Check sheet for the modelled part. Datum: model origin and axes. Units: mm. Face numbers are marked on the shaded views. Round coordinates to 2 decimals unless told otherwise and drop trailing zeros. Loops run counter-clockwise (first coordinate to the right, second up) from the corner with the lowest first, then second, coordinate; pieces in that order, holes last. Notation, with made-up numbers: M 76.5,11.25 L 122.5,11.25 A16 cw 122.5,36.25 Z; hole C -28.75,-26 d2. An arc over 180 degrees is marked long. One line per question, with ' | ' between items. Start each with the question number.
(1) Section check B-B (y = 3). Record the boundary of the cut face in (x, z).
(2) Section check C-C (x = -7.25). Record the boundary of the cut face in (y, z).
(3) Thickness scan on probe 1 along Y at (x, z) = (-9, 14.25); probe 2 along Y at (x, z) = (-7, 7.25); probe 3 along X at (y, z) = (3.75, 7). Record the ranges inside material, lowest first. Write a range as [from, to].
(4) Draft check along X on the marked faces 1, 2 and 3. Enter one of: +X half, -X half, draft (parallel to the pull), parting line (faces both ways), or undercut.
(5) Go/stop test with flat-tipped pins: P1, Ø5, axis at x = -8, z = 10.5, coming from the +Y side; P2, Ø6, axis at x = 3.5, z = 8, coming from the +Y side; P3, Ø5, axis at y = 17.5, z = 3, coming from the -X side. Record where each tip stops, or that it passes through.
```python
from build123d import *

# Parameters (mm, degrees)
CYLINDER001_R     = 1.5
CYLINDER001_DEPTH = 40
ARRAY_COUNT       = 8
CYLINDER_R        = 10
CYLINDER_DEPTH    = 15


with BuildPart() as array:
    # Cylinder001 → Cylinder001 (new body)
    with BuildSketch(Plane.XY):
        Circle(CYLINDER001_R)
    extrude(amount=CYLINDER001_DEPTH)

    # Array: Array ×8 about axis
    array_axis = Axis((0, 10, 0), (0, 0, 1))


with BuildPart() as array_1:
    add(array.part)
    for i in range(1, ARRAY_COUNT):
        add(array.part.rotate(array_axis, i * 360 / ARRAY_COUNT))


with BuildPart() as cut:
    # Cylinder → Cylinder (new body)
    with BuildSketch(Plane(origin=(0, 10, 0), x_dir=(1, 0, 0), z_dir=(0, 0, 1))):
        Circle(CYLINDER_R)
    extrude(amount=CYLINDER_DEPTH)

    # Cut: cut Array
    add(array_1.part, mode=Mode.SUBTRACT)


solid = cut.part
```
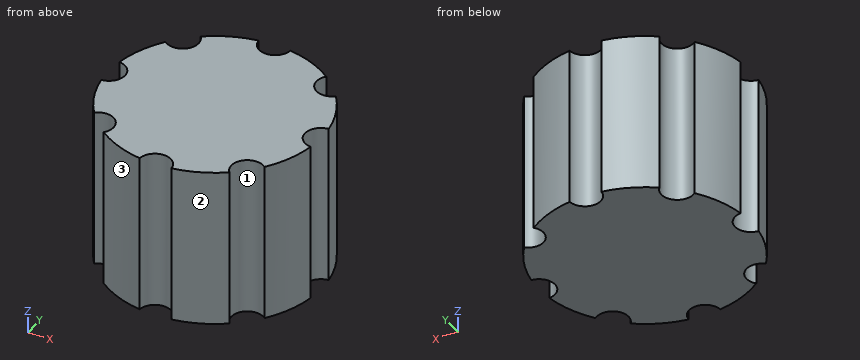
The answers:
1) outline: M -5.57,0 L 5.57,0 L 5.57,15 L -5.57,15 Z
2) outline: M 4.42,0 L 15.58,0 L 15.58,15 L 4.42,15 Z
3) probe 1: [5.64, 8.88], [11.12, 14.36] | probe 2: [4.43, 15.57] | probe 3: [-5.82, 5.82]
4) face 1: undercut | face 2: +X half | face 3: -X half
5) P1: y = 18.35 | P2: y = 19.89 | P3: x = -8.66
